from build123d import *

# Parameters (mm, degrees)
SKETCH1_R           = 12.75
SKETCH1_R_2         = 3.175
BOSS_EXTRUDE2_DEPTH = 8
BOSS_EXTRUDE3_DEPTH = 66
SKETCH4_R           = 1.6
CUT_EXTRUDE1_DEPTH  = 6
CUT_EXTRUDE2_DEPTH  = 62
BOSS_EXTRUDE4_DEPTH = 10
CUT_EXTRUDE3_START  = -66
CUT_EXTRUDE3_DEPTH  = 66


with BuildPart() as part:
    # Sketch1 → Boss-Extrude2 (new body)
    with BuildSketch(Plane(origin=(0, 0, 0), x_dir=(1, 0, 0), z_dir=(0, 1, 0))):
        with BuildLine():
            Line((0, 16.75), (-16.278174593, 20.278174593))
            ThreePointArc((-16.278174593, 20.278174593), (-26.52081528, 24.52081528), (-22.278174593, 14.278174593))
            Line((-22.278174593, 14.278174593), (-19.5, 0))
            Line((-19.5, 0), (-22.278174593, -14.278174593))
            ThreePointArc((-22.278174593, -14.278174593), (-26.52081528, -24.52081528), (-16.278174593, -20.278174593))
            Line((-16.278174593, -20.278174593), (0, -16.75))
            ThreePointArc((0, -16.75), (7.9526392, -14.741710543), (13.998269272, -9.198421462))
            Line((13.998269272, -9.198421462), (23.25, -6.5))
            ThreePointArc((23.25, -6.5), (29.75, 0), (23.25, 6.5))
            Line((23.25, 6.5), (13.998269272, 9.198421462))
            ThreePointArc((13.998269272, 9.198421462), (7.9526392, 14.741710543), (0, 16.75))
        make_face()
        with Locations(Location((0, 0, 0), (0, 0, 270))):
            Circle(SKETCH1_R, mode=Mode.SUBTRACT)
        with Locations(Location((23.25, 0, 0), (0, 0, 270))):
            Circle(SKETCH1_R_2, mode=Mode.SUBTRACT)
        with Locations(Location((-22.278174593, 20.278174593, 0), (0, 0, 270))):
            Circle(SKETCH1_R_2, mode=Mode.SUBTRACT)
        with Locations(Location((-22.278174593, -20.278174593, 0), (0, 0, 90))):
            Circle(SKETCH1_R_2, mode=Mode.SUBTRACT)
    extrude(amount=BOSS_EXTRUDE2_DEPTH)

    # Sketch2 → Boss-Extrude3 (add)
    with BuildSketch(Plane(origin=(0, 8, 0), x_dir=(1, 0, 0), z_dir=(0, 1, 0))):
        with BuildLine():
            Line((-7.607743292, -18.398922392), (0, -16.75))
            ThreePointArc((0, -16.75), (7.9526392, -14.741710543), (13.998269272, -9.198421462))
            Line((13.998269272, -9.198421462), (15.058663133, -6.806802563))
            ThreePointArc((15.058663133, -6.806802563), (16.5, 0), (15.058663133, 6.806802563))
            Line((15.058663133, 6.806802563), (13.998269272, 9.198421462))
            ThreePointArc((13.998269272, 9.198421462), (7.9526392, 14.741710543), (0, 16.75))
            Line((0, 16.75), (-7.607743292, 18.398922392))
            ThreePointArc((-7.607743292, 18.398922392), (-12.83286117, 18.130965758), (-17.207513674, 15.261109827))
            ThreePointArc((-17.207513674, 15.261109827), (-17.954443829, 14.374906845), (-18.65578326, 13.452202458))
            ThreePointArc((-18.65578326, 13.452202458), (-18.894540484, 13.105967779), (-19.118527996, 12.75))
            Line((-19.118527996, 12.75), (-19.118527996, -12.75))
            ThreePointArc((-19.118527996, -12.75), (-18.894540484, -13.105967779), (-18.65578326, -13.452202458))
            ThreePointArc((-18.65578326, -13.452202458), (-17.954443829, -14.374906845), (-17.207513674, -15.261109827))
            ThreePointArc((-17.207513674, -15.261109827), (-12.83286117, -18.130965758), (-7.607743292, -18.398922392))
        make_face()
        with BuildLine():
            Line((-15, 12.75), (-15, -12.75))
            Line((-15, -12.75), (-12.75, -12.75))
            Line((-12.75, -12.75), (-12.75, -8.75))
            ThreePointArc((-12.75, -8.75), (-12.457106781, -8.042893219), (-11.75, -7.75))
            Line((-11.75, -7.75), (-10.124228366, -7.75))
            ThreePointArc((-10.124228366, -7.75), (12.75, 0), (-10.124228366, 7.75))
            Line((-10.124228366, 7.75), (-11.5, 7.75))
            ThreePointArc((-11.5, 7.75), (-12.207106781, 8.042893219), (-12.5, 8.75))
            Line((-12.5, 8.75), (-12.5, 12.75))
            Line((-12.5, 12.75), (-15, 12.75))
        make_face(mode=Mode.SUBTRACT)
    extrude(amount=BOSS_EXTRUDE3_DEPTH)

    # Sketch4 → Cut-Extrude1 (cut)
    with BuildSketch(Plane.ZY.offset(19.118527996)):
        with Locations((10.95, 66.47)):
            Circle(SKETCH4_R)
        with Locations(Location((-10.95, 66.47, 0), (0, 0, 180))):
            Circle(SKETCH4_R)
        with Locations((10.95, 34.72)):
            Circle(SKETCH4_R)
        with Locations(Location((-10.95, 34.72, 0), (0, 0, 180))):
            Circle(SKETCH4_R)
    extrude(amount=-CUT_EXTRUDE1_DEPTH, mode=Mode.SUBTRACT)

    # Sketch5 → Cut-Extrude2 (cut)
    with BuildSketch(Plane(origin=(-15, 0, 0), x_dir=(0, 0, -1), z_dir=(1, 0, 0))):
        Polygon((-5, 17), (-7, 17), (-7, 20), (0, 20), (11, 20), (11, 17), (9, 17), (9, 11), (0, 11), (-5, 11), align=None)
    extrude(amount=CUT_EXTRUDE2_DEPTH, mode=Mode.SUBTRACT)

    # Sketch6 → Boss-Extrude4 (add)
    with BuildSketch(Plane(origin=(-15, 0, 0), x_dir=(0, 0, -1), z_dir=(1, 0, 0))):
        Polygon((11, 20), (11, 17), (9, 17), (9, 11), (6.130608727, 11), (6.130608727, 20), align=None)
    extrude(amount=BOSS_EXTRUDE4_DEPTH)

    # Sketch7 → Cut-Extrude3 (cut)
    with BuildSketch(Plane(origin=(0, 74, 0), x_dir=(1, 0, 0), z_dir=(0, 1, 0)).offset(CUT_EXTRUDE3_START)):
        with BuildLine():
            Line((-15, 12.75), (-15, 4.5))
            Line((-15, 4.5), (-3.997712125, 4.5))
            Line((-3.997712125, 4.5), (-3.997712125, 12.107055702))
            ThreePointArc((-3.997712125, 12.107055702), (-7.389403522, 10.39034242), (-10.124228366, 7.75))
            Line((-10.124228366, 7.75), (-11.5, 7.75))
            ThreePointArc((-11.5, 7.75), (-12.207106781, 8.042893219), (-12.5, 8.75))
            Line((-12.5, 8.75), (-12.5, 12.75))
            Line((-12.5, 12.75), (-15, 12.75))
        make_face()
    extrude(amount=CUT_EXTRUDE3_DEPTH, mode=Mode.SUBTRACT)


solid = part.part
Verification items for the finished model (mm, model axes). A direction names the side the tool comes from. Coordinates: 2 decimals unless noted, no trailing zeros. Order: outer loops, then holes, each group sorted by start corner. A loop starts at its lowest first (then second) coordinate and runs counter-clockwise, first axis right, second up. Notation, with made-up numbers: (31, -19) -> (50, -19) arc R21 ccw to (50, 18) -> close; hole circle Ø5 at (63, 58). An arc over 180 degrees is marked (long way). Put each result on its own line as item: value. Start each with the question number.
1. Material ranges on L1, parallel to Y at x = -17.05, z = -10.95; L2, parallel to X at y = 2.75, z = 0 (3 decimals); L3, parallel to Z at x = 14, y = 14, recorded low to high. Write a range as [from, to].
2. Cross-section at D-D, the plane y = 19. Record the boundary of the cut face in (x, z), then the cut area to 3 significant figures.
3. Access from +Z, -Z, +X, -X, +Y, -Y to the whole of each face (thin tool, end or side, straight path). Record for faces 1 (the cylindrical face through (-17.965, 40.538, 14.362)), 2 (the flat face through (14.52, 40.54, 8.02)), 3 (the flat face through (-15, 41, 0)), 4 (the cylindrical face through (-17.09, 65.05, 11.69)).
4. Cross-section at C-C, the plane z = 10.95. Record the boundary of the cut face in (x, y).
5. Cross-section at A-A, the plane y = 5. Record the boundary of the cut face in (x, z) (3 decimals).
6. Go/stop test with flat-tipped pins: pin 1 Ø4 at (x, y) = (-17.5, 26) entering from -Z; pin 2 Ø6 at (x, z) = (-23, -12.5) entering from +Y; pin 3 Ø4 at (x, z) = (-22.28, -20.28) entering from -Y; pin 4 Ø6 at (y, z) = (62.5, -3) entering from -X. Record where each tip stops, or that it passes through.
7. Mould release check, pull along X, two halves, no side actions. Record for faces 5 (the cylindrical face through (-17.94, 40.54, -14.39)), 6 (the cylindrical face through (16.42, 10.44, 1.65)), 7 (the flat face through (-11, 41, 7.75)), 8 (the flat face through (-12.5, 41, -11)): released by +X, released by -X, zero draft, split by the parting line, or undercut.
Computed:
1. L1: [0, 33.12], [36.32, 64.87], [68.07, 74]
1. L2: [-19.5, -12.75], [12.75, 20.075], [26.425, 29.75]
1. L3: [-9.19, -9], [5, 9.19]
2. outline: (-19.12, -12.75) arc R10 ccw to (-18.66, -13.45) arc R23 ccw to (-17.21, -15.26) arc R10 ccw to (-7.61, -18.4) -> (0, -16.75) arc R16.75 ccw to (12.63, -11) -> (6.45, -11) arc R12.75 cw to (-10.12, -7.75) -> (-11.5, -7.75) arc R1 ccw to (-12.5, -8.75) -> (-12.5, -12.75) -> (-15, -12.75) -> (-15, 12.75) -> (-12.75, 12.75) -> (-12.75, 8.75) arc R1 ccw to (-11.75, 7.75) -> (-10.12, 7.75) arc R12.75 cw to (10.66, 7) -> (14.97, 7) -> (14, 9.2) arc R16.75 ccw to (0, 16.75) -> (-7.61, 18.4) arc R10 ccw to (-17.21, 15.26) arc R23 ccw to (-18.66, 13.45) arc R10 ccw to (-19.12, 12.75) -> close
2. area: 442 mm2
3. face 1: +Z, -X, +Y
3. face 2: +Z, +X, +Y
3. face 3: +Y
3. face 4: -X
4. outline: (-21.63, 0) -> (-6.53, 0) -> (-6.53, 74) -> (-12.75, 74) -> (-12.75, 8) -> (-15, 8) -> (-15, 33.12) -> (-19.12, 33.12) -> (-19.12, 8) -> (-21.63, 8) -> close; (-19.12, 36.32) -> (-15, 36.32) -> (-15, 64.87) -> (-19.12, 64.87) -> close; (-19.12, 68.07) -> (-15, 68.07) -> (-15, 74) -> (-19.12, 74) -> close; (6.53, 0) -> (12.68, 0) -> (12.68, 74) -> (6.53, 74) -> close
5. outline: (-22.278, -14.278) arc R6 ccw (long way) to (-16.278, -20.278) -> (0, -16.75) arc R16.75 ccw to (13.998, -9.198) -> (23.25, -6.5) arc R6.5 ccw to (23.25, 6.5) -> (13.998, 9.198) arc R16.75 ccw to (0, 16.75) -> (-16.278, 20.278) arc R6 ccw (long way) to (-22.278, 14.278) -> (-19.5, 0) -> close; hole circle Ø6.35 at (-22.278, -20.278); hole circle Ø6.35 at (-22.278, 20.278); hole circle Ø25.5 at (0, 0); hole circle Ø6.35 at (23.25, 0)
6. pin 1: z = -16.79
6. pin 2: y = 8
6. pin 3: through
6. pin 4: x = -19.12
7. face 5: released by -X
7. face 6: released by +X
7. face 7: undercut
7. face 8: undercut
